```python
from build123d import *

# Parameters (mm, degrees)
F1_DEPTH = 75
F3_D     = 4.1
F2_W     = 60
F2_H     = 17
F4_DEPTH = 11
F5_R     = 4
F6_R     = 2


with BuildPart() as f1:
    # F0 (on Front) → F1 (new body)
    with BuildSketch(Plane.XZ):
        Polygon((-19.3604914132, 7.6604444312), (-12.9326153163, 0), (0, 0), (0, 17), (-2, 17), (-2, 2), (-12, 2), (-12, 8.1604444312), (-19.3604914132, 8.1604444312), align=None)
    extrude(amount=F1_DEPTH)

    # F3 (through all)
    with Locations(Plane.YZ):
        with Locations((-67.5, 12)):
            Hole(F3_D / 2)

    # F2 (on face) → F4 (cut)
    with BuildSketch(Plane.YZ):
        with Locations((-30, 8.5)):
            Rectangle(F2_W, F2_H)
    extrude(amount=-F4_DEPTH, mode=Mode.SUBTRACT)

    # F5
    f5_edges = [f1.edges().sort_by_distance(p)[0] for p in [
        (-11, -60, 1),
    ]]
    fillet(f5_edges, radius=F5_R)

    # F6
    f6_edges = [f1.edges().sort_by_distance(p)[0] for p in [
        (-1, -60, 17),
        (-1, -75, 17),
    ]]
    fillet(f6_edges, radius=F6_R)

    # F7: F1 across face


with BuildPart() as f1_1:
    add(f1.part)
    add(f1.part.mirror(Plane(origin=(-14.4459717542, 0, 4.9195457807), x_dir=(1, 0, 0), z_dir=(0, 1, 0))))


solid = f1_1.part
```
The listing builds one solid part. Answer for the finished solid, in the listing's coordinates (mm). A direction names the side the tool comes from. Coordinates: 2 decimals unless noted, no trailing zeros. Write each loop counter-clockwise with the first axis right and the second up, starting at its lowest first coordinate (ties: lowest second). Pieces come first, ordered by that corner, then holes. Notation, with made-up numbers: (50.5, 15) - (54.5, 15) arc R15 cw to (54.5, 38) - close; hole circle Ø1 at (-21, 7). An arc over 180 degrees is marked (long way). Return JSON: item names as keys, results as strings. Group by question number.
1. A cutting plane is placed at D-D, the plane x = -15.25. Determine the outline of the cut face in (y, z), plus the area to 3 significant figures.
2. A cutting plane is placed at C-C, the plane z = 5. Determine the outline of the cut face in (x, y), plus the area to 3 significant figures.
3. Straight lines are drawn through the part: L1, parallel to Z at x = -1.25, y = -67.5; L2, parallel to Y at x = -1, z = 8; L3, parallel to X at y = -64, z = 14.5. For each, find the intervals that lie inside material, in ascending order.
4. A cutting plane is placed at A-A, the plane y = -67.5. Determine the outline of the cut face in (x, z), plus the area to 3 significant figures.
5. Which of the six approach directions +Z, -Z, +X, -X, +Y, -Y give full straight-line access (tool end or side, diameter ignored) to faces 1 (the flat face through (-12, -1, 5)), 2 (the flat face through (-8, -75, 1)), 3 (the flat face through (-16, -1, 8.16)), 4 (the cylindrical face through (-9.859, -58.797, 1.014))?
6. Given pin 1 (10 mm diameter, centred on x = -10, y = 49.5, fed in from +Z); pin 2 (7 mm diameter, centred on y = 23.5, z = 5, fed in from +X); pin 3 (3 mm diameter, centred on x = -11.5, y = -35.5, fed in from -Z), each flat-ended and moving along its own axis, determine where each tip first touches the part or whether it passes through.
7. A cutting plane is placed at B-B, the plane z = 12. Determine the outline of the cut face in (x, y).
8. Determine the mould class of faces 5 (the flat face through (-2, -67.4, 9.6)), 6 (the flat face through (-8, 75, 1)), 7 (the cylindrical face through (-9.859, 58.797, 1.014)) for opening direction Y: released by +Y, released by -Y, zero draft, split by the parting line, or undercut.
Ans:
{
 "1": {"outline": "(-75, 2.76) - (75, 2.76) - (75, 8.16) - (-75, 8.16) - close", "area": "810 mm²"},
 "2": {"outline": "(-17.13, -75) - (-12, -75) - (-12, 75) - (-17.13, 75) - close; (-2, -75) - (0, -75) - (0, -60) - (-2, -60) - close; (-2, 60) - (0, 60) - (0, 75) - (-2, 75) - close", "area": "829 mm²"},
 "3": {"L1": "0 to 9.95, 14.05 to 17", "L2": "-75 to -60, 60 to 75", "L3": "-2 to 0"},
 "4": {"outline": "(-19.36, 7.66) - (-12.93, 0) - (0, 0) - (0, 9.95) - (-2, 9.95) - (-2, 2) - (-12, 2) - (-12, 8.16) - (-19.36, 8.16) - close; (-2, 14.05) - (0, 14.05) - (0, 17) - (-2, 17) - close", "area": "81.2 mm²"},
 "5": {"face 1": "+Z, +Y, -Y", "face 2": "+Z, -Z, +X, -X, -Y", "face 3": "+Z, -X, +Y, -Y", "face 4": "+Z, -Z, +X"},
 "6": {"pin 1": "z = 8.16", "pin 2": "x = -11", "pin 3": "z = 0"},
 "7": {"outline": "(-2, -75) - (0, -75) - (0, -69.55) - (-2, -69.55) - close; (-2, -65.45) - (0, -65.45) - (0, -60) - (-2, -60) - close; (-2, 60) - (0, 60) - (0, 65.45) - (-2, 65.45) - close; (-2, 69.55) - (0, 69.55) - (0, 75) - (-2, 75) - close"},
 "8": {"face 5": "zero draft", "face 6": "released by +Y", "face 7": "undercut"}
}
